For this review, use the dimensioned drawing (mm, ordinates from the lowest corner) and the shaded views. Round coordinates to 2 decimals unless told otherwise and drop trailing zeros. Loops run counter-clockwise (first coordinate to the right, second up) from the corner with the lowest first, then second, coordinate; pieces in that order, holes last. Notation, with made-up numbers: M 19.5,33.25 L 72.5,33.25 A21 cw 72.5,61.25 Z; hole C 1.5,82 d10. An arc over 180 degrees is marked long. Answer as a JSON object with one key per item and string values. Group by question number.
Item 1: Consider section A-A (z = 80.9). Give the boundary of the cut face in (x, y), and give its area (3 significant figures).
Item 2: Consider section B-B (x = 3). Give the boundary of the cut face in (y, z).
Item 3: Consider section C-C (z = 8). Give the boundary of the cut face in (x, y), and give its area (3 significant figures).
Item 4: Insertion check: P1, Ø2.5, axis at x = 3, z = 119.1, coming from the +Y side; P2, Ø4, axis at x = 22.5, y = 10, coming from the -Z side. Each pin has a flat end and moves straight along its axis. Give the tip position at first contact, or say it passes through.
Item 5: To check wall thickness, follow line 1 (X direction, y = 10, z = 6.5); line 2 (Y direction, x = 7.5, z = 4.25); line 3 (X direction, y = 14.5, z = 119.1). State the ranges of each line that lie inside material, in increasing order.
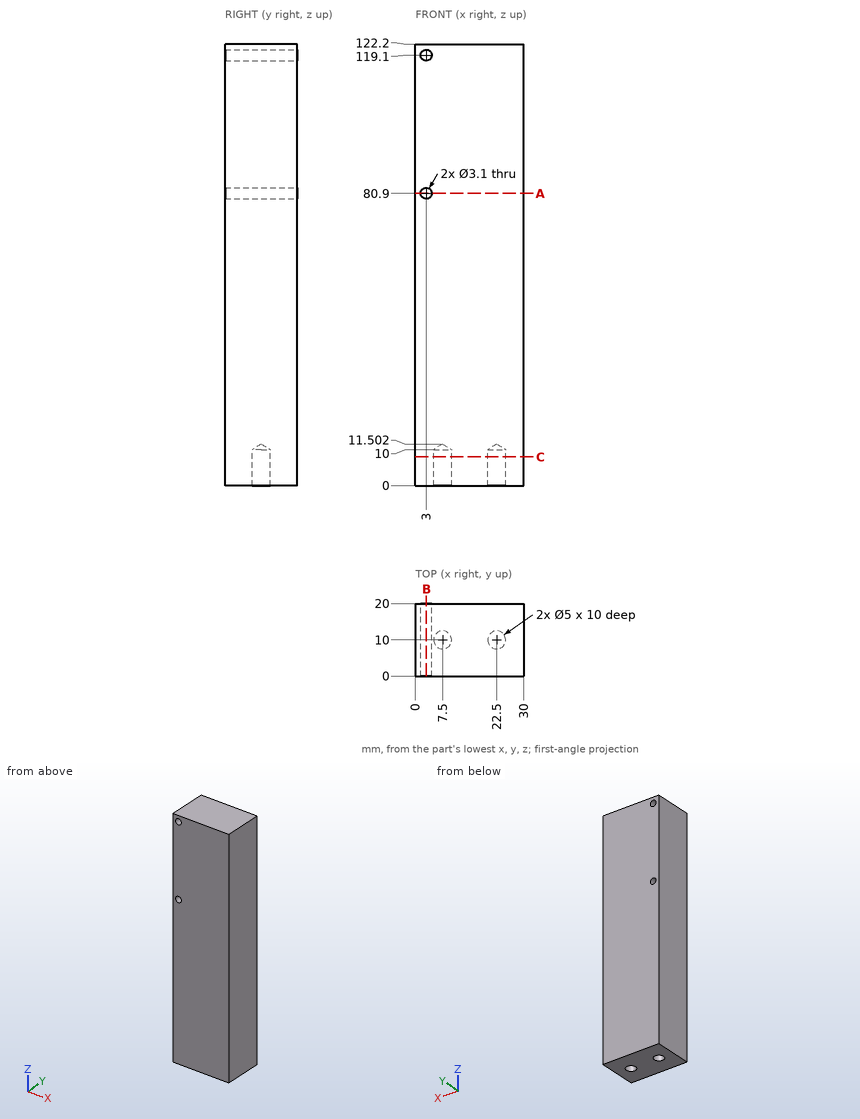
Geometry results:
{
 "1": {"outline": "M 0,0 L 1.45,0 L 1.45,20 L 0,20 Z; M 4.55,0 L 30,0 L 30,20 L 4.55,20 Z", "area": "538 mm^2"},
 "2": {"outline": "M 0,0 L 20,0 L 20,79.35 L 0,79.35 Z; M 0,82.45 L 20,82.45 L 20,117.55 L 0,117.55 Z; M 0,120.65 L 20,120.65 L 20,122.2 L 0,122.2 Z"},
 "3": {"outline": "M 0,0 L 30,0 L 30,20 L 0,20 Z; hole C 7.5,10 d5; hole C 22.5,10 d5", "area": "561 mm^2"},
 "4": {"P1": "passes through", "P2": "stops at z = 10.3"},
 "5": {"line 1": "x = 0 to 5, 10 to 20, 25 to 30", "line 2": "y = 0 to 7.5, 12.5 to 20", "line 3": "x = 0 to 1.45, 4.55 to 30"}
}
